Read the model definition and answer for the solid it produces. Units are mm, in the model's axes. Round coordinates to 2 decimals unless told otherwise and drop trailing zeros. Loops run counter-clockwise (first coordinate to the right, second up) from the corner with the lowest first, then second, coordinate; pieces in that order, holes last. Notation, with made-up numbers: (22, -12) -> (78, -12) arc R21 ccw to (78, 26) -> close; hole circle Ø5 at (35, 74). An arc over 180 degrees is marked (long way). Put each result on its own line as item: value.
from build123d import *

# Parameters (mm, degrees)
SKETCH_1_R   = 7.5
SKETCH_1_R_2 = 5.7


with BuildPart() as part:
    # 扫描1: sweep along a path in 草图2
    with BuildLine(Plane(origin=(0, 0, 0), x_dir=(1, 0, 0), z_dir=(0, 1, 0))) as sweep_1_path:
        Line((0, 0), (20, 0))
        ThreePointArc((20, 0), (40, 20), (20, 40))
        Line((20, 40), (0, 40))
    # 草图1 → 扫描1 (sweep)
    with BuildSketch(Plane(origin=(0, 0, 0), x_dir=(0, 0, -1), z_dir=(1, 0, 0))):
        Circle(SKETCH_1_R)
        Circle(SKETCH_1_R_2, mode=Mode.SUBTRACT)
    sweep(path=sweep_1_path.line)


solid = part.part
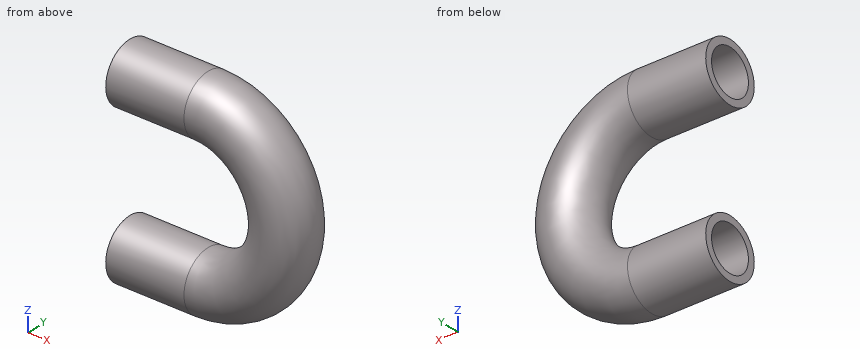
Item 1: The part is cut by section D-D (x = 28.5). State how many separate pieces and enclosed holes the cut face has, then the cut area to 3 significant figures.
Derived:
separate pieces: 2
enclosed holes: 2
area: 170 mm^2
Item 2: The part is cut by section C-C (y = 6.5). Determine the outline of the cut face in (x, z), then the cut area to 3 significant figures.
Derived:
outline: (0, -43.74) -> (20, -43.74) arc R23.74 ccw to (20, 3.74) -> (0, 3.74) -> (0, -3.74) -> (20, -3.74) arc R16.26 cw to (20, -36.26) -> (0, -36.26) -> close
area: 770 mm^2
Item 3: The part is cut by section B-B (x = 18). Determine the outline of the cut face in (y, z), then the cut area to 3 significant figures.
Derived:
outline: circle Ø15 at (0, -40); circle Ø15 at (0, 0); hole circle Ø11.4 at (0, -40); hole circle Ø11.4 at (0, 0)
area: 149 mm^2
Item 4: Flat-ended cylindrical pins translate along their axes: pin 1 Ø5 at (y, z) = (5, -13.5) entering from +X; pin 2 Ø1 at (x, y) = (33, -3) entering from +Z; pin 3 Ø3 at (y, z) = (4.5, -34) entering from +X; pin 4 Ø12 at (x, z) = (36, -25.5) entering from +Y. Find the tip coordinate at first contact, or state that the pin passes through.
Derived:
pin 1: stops at x = 46.43
pin 2: stops at z = 3.88
pin 3: stops at x = 43.32
pin 4: stops at y = 7.5
Item 5: The part is cut by section A-A (y = -3.5). Determine the outline of the cut face in (x, z), then the cut area to 3 significant figures.
Derived:
outline: (0, -46.63) -> (20, -46.63) arc R26.63 ccw to (20, 6.63) -> (0, 6.63) -> (0, 4.5) -> (20, 4.5) arc R24.5 cw to (20, -44.5) -> (0, -44.5) -> close; (0, -35.5) -> (20, -35.5) arc R15.5 ccw to (20, -4.5) -> (0, -4.5) -> (0, -6.63) -> (20, -6.63) arc R13.37 cw to (20, -33.37) -> (0, -33.37) -> close
area: 439 mm^2
Item 6: Find the intervals of material crossed by line 1 along Z through (x, y) = (32.5, -4.25); line 2 along Y through (x, z) = (37, -9); line 3 along Z through (x, y) = (3, -4.75), in increasing order.
Derived:
line 1: z = -43 to -40.25, -30.31 to -25.9, -14.1 to -9.69, 0.25 to 3
line 2: y = -7.5 to -5.69, 5.69 to 7.5
line 3: z = -45.8 to -43.15, -36.85 to -34.2, -5.8 to -3.15, 3.15 to 5.8
